The model under review builds one solid part; all positions refer to its coordinate system, in mm. Coordinates: 2 decimals unless noted, no trailing zeros. Write each loop counter-clockwise with the first axis right and the second up, starting at its lowest first coordinate (ties: lowest second). Pieces come first, ordered by that corner, then holes. Notation, with made-up numbers: (1, -16.75) - (18, -16.75) arc R12 ccw to (18, 5.25) - close; hole circle Ø9 at (49.25, -11.75). An arc over 180 degrees is marked (long way). Put each result on its own line as item: value.
Autodesk Fusion 360 part; units mm, degrees
sketch "Sketch1" plane through (0, 0, 0) normal (0, 1, 0) x (1, 0, 0)
  line L0 (7.9, 2.9) -> (7.9, 4.9)
  line L1 (-2.7515, -3.6) -> (-4.9, -5.7485)
  line L2 (2.9, -7.9) -> (4.9, -7.9)
  line L3 (-2.9, -7.9) -> (-2.9, -10.1)
  arc A0 (-10.1, -9) -> (-9, -10.1) centre (-9, -9) ccw
  line L4 (5.7485, 4.9) -> (3.6, 2.7515)
  line L5 (-7.9, 2.9) -> (-10.1, 2.9)
  line L6 (-4.9, -7.9) -> (-2.9, -7.9)
  line L7 (4.9, 5.7485) -> (4.9, 7.9)
  line L8 (10.1, 2.9) -> (7.9, 2.9)
  line L9 (9, -10.1) -> (2.9, -10.1)
  arc A1 (9, -10.1) -> (10.1, -9) centre (9, -9) ccw
  line L10 (4.9, -5.7485) -> (2.7515, -3.6)
  line L11 (5.7485, -4.9) -> (7.9, -4.9)
  line L12 (-10.1, 2.9) -> (-10.1, 9)
  line L13 (7.9, -2.9) -> (10.1, -2.9)
  line L14 (-3.6, 2.7515) -> (-5.7485, 4.9)
  line L15 (10.1, -2.9) -> (10.1, -9)
  line L16 (-2.9, 10.1) -> (-2.9, 7.9)
  line L17 (7.9, -4.9) -> (7.9, -2.9)
  line L18 (-3.6, -2.7515) -> (-3.6, 2.7515)
  line L19 (3.6, 2.7515) -> (3.6, -2.7515)
  line L20 (2.7515, -3.6) -> (-2.7515, -3.6)
  line L21 (-10.1, -9) -> (-10.1, -2.9)
  line L22 (10.1, 9) -> (10.1, 2.9)
  line L23 (2.9, 7.9) -> (2.9, 10.1)
  line L24 (7.9, 4.9) -> (5.7485, 4.9)
  line L25 (-2.9, -10.1) -> (-9, -10.1)
  line L26 (-2.7515, 3.6) -> (2.7515, 3.6)
  arc A2 (-9, 10.1) -> (-10.1, 9) centre (-9, 9) ccw
  line L27 (4.9, 7.9) -> (2.9, 7.9)
  line L28 (-7.9, -4.9) -> (-5.7485, -4.9)
  line L29 (2.9, 10.1) -> (9, 10.1)
  arc A3 (10.1, 9) -> (9, 10.1) centre (9, 9) ccw
  line L30 (-4.9, -5.7485) -> (-4.9, -7.9)
  line L31 (-7.9, -2.9) -> (-7.9, -4.9)
  line L32 (-4.9, 7.9) -> (-4.9, 5.7485)
  line L33 (2.7515, 3.6) -> (4.9, 5.7485)
  line L34 (-4.9, 5.7485) -> (-2.7515, 3.6)
  line L35 (-10.1, -2.9) -> (-7.9, -2.9)
  line L36 (3.6, -2.7515) -> (5.7485, -4.9)
  line L37 (4.9, -7.9) -> (4.9, -5.7485)
  line L38 (2.9, -10.1) -> (2.9, -7.9)
  line L39 (-5.7485, -4.9) -> (-3.6, -2.7515)
  line L40 (-7.9, 4.9) -> (-7.9, 2.9)
  line L41 (-2.9, 7.9) -> (-4.9, 7.9)
  line L42 (-9, 10.1) -> (-2.9, 10.1)
  line L43 (-5.7485, 4.9) -> (-7.9, 4.9)
  line L44 (-15.1, -14.6) -> (13.1, -14.6)
  line L45 (13.1, -14.6) -> (13.1, 14.6)
  line L46 (13.1, 14.6) -> (-15.1, 14.6)
  line L47 (-15.1, 14.6) -> (-15.1, -14.6)
  dimension "d1" = 3
  dimension "d2" = 5
  dimension "d3" = 4.5
  dimension "d4" = 4.5
extrude "Extrude1" add sketch "Sketch1" along normal blind 3 contours L0 L1 L2 L3 A0 L4 L5 L6 L7 L8 L9 A1 L10 L11 L12 L13 L14 L15 L16 L17 L18 L19 L20 L21 L22 L23 L24 L25 L26 A2 L27 L28 L29 A3 L30 L31 L32 L33 L34 L35 L36 L37 L38 L39 L40 L41 L42 L43 | L44 L45 L46 L47
extrude "Extrude2" add sketch "Sketch1" along normal blind 30 from surface at 3
mirror "Mirror1" about plane through (-15.1, 3, -14.6) normal (-1, 0, 0) of bodies 1 merged
ref_plane "WorkPlane1" through (-15.1, 16.5, -44.6) normal (0, 0, -1) x (-1, 0, 0)
sketch "Sketch2" plane through (0, 0, -44.6) normal (0, 0, -1) x (-1, 0, 0)
  line L0 (-13.1, 0) -> (43.3, 0)
  line L1 (43.3, 0) -> (43.3, 33)
  line L2 (43.3, 33) -> (-13.1, 33)
  line L3 (-13.1, 33) -> (-13.1, 0)
  line L4 (28.1, 33) -> (2.1, 33)
  line L5 (2.1, 33) -> (2.1, 7)
  line L6 (2.1, 7) -> (28.1, 7)
  line L7 (28.1, 7) -> (28.1, 33)
  line L8 (15.1, 33) -> (15.1, 0) construction
  line L9 (25.3, 30.2) -> (4.9, 30.2)
  line L10 (4.9, 30.2) -> (4.9, 9.8)
  line L11 (4.9, 9.8) -> (25.3, 9.8)
  line L12 (25.3, 9.8) -> (25.3, 30.2)
  dimension "d15" = 20.4
  dimension "d17" = 2.8
  dimension "d18" = 2.8
  dimension "d29" = 2.8
loft "Loft1" add profiles "Sketch2" section 1 face at (-5.7, 11, -14.6) section 2 contours L2 L4 L5 L6 L7 | L9 L10 L11 L12
extrude "Extrude3" cut sketch "Sketch2" against normal blind 30 contours L9 L10 L11 L12
sketch "Sketch3" plane through (0, 33, 0) normal (0, 1, 0) x (-1, 0, 0)
  line L0 (21.2, 10.1) -> (27.3, 10.1)
  line L1 (27.3, 10.1) -> (27.3, 7.9)
  line L2 (27.3, 7.9) -> (25.3, 7.9)
  line L3 (25.3, 7.9) -> (25.3, 5.7485)
  line L4 (25.3, 5.7485) -> (27.4485, 3.6)
  line L5 (27.4485, 3.6) -> (32.9515, 3.6)
  line L6 (32.9515, 3.6) -> (35.1, 5.7485)
  line L7 (35.1, 5.7485) -> (35.1, 7.9)
  line L8 (35.1, 7.9) -> (33.1, 7.9)
  line L9 (33.1, 7.9) -> (33.1, 10.1)
  line L10 (33.1, 10.1) -> (39.2, 10.1)
  arc A0 (40.3, 9) -> (39.2, 10.1) centre (39.2, 9) ccw
  line L11 (40.3, 9) -> (40.3, 2.9)
  line L12 (40.3, 2.9) -> (38.1, 2.9)
  line L13 (38.1, 2.9) -> (38.1, 4.9)
  line L14 (38.1, 4.9) -> (35.9485, 4.9)
  line L15 (35.9485, 4.9) -> (33.8, 2.7515)
  line L16 (33.8, 2.7515) -> (33.8, -2.7515)
  line L17 (33.8, -2.7515) -> (35.9485, -4.9)
  line L18 (35.9485, -4.9) -> (38.1, -4.9)
  line L19 (38.1, -4.9) -> (38.1, -2.9)
  line L20 (38.1, -2.9) -> (40.3, -2.9)
  line L21 (40.3, -2.9) -> (40.3, -9)
  arc A1 (39.2, -10.1) -> (40.3, -9) centre (39.2, -9) ccw
  line L22 (39.2, -10.1) -> (33.1, -10.1)
  line L23 (33.1, -10.1) -> (33.1, -7.9)
  line L24 (33.1, -7.9) -> (35.1, -7.9)
  line L25 (35.1, -7.9) -> (35.1, -5.7485)
  line L26 (35.1, -5.7485) -> (32.9515, -3.6)
  line L27 (32.9515, -3.6) -> (27.4485, -3.6)
  line L28 (27.4485, -3.6) -> (25.3, -5.7485)
  line L29 (25.3, -5.7485) -> (25.3, -7.9)
  line L30 (25.3, -7.9) -> (27.3, -7.9)
  line L31 (27.3, -7.9) -> (27.3, -10.1)
  line L32 (27.3, -10.1) -> (21.2, -10.1)
  arc A2 (20.1, -9) -> (21.2, -10.1) centre (21.2, -9) ccw
  line L33 (20.1, -9) -> (20.1, -2.9)
  line L34 (20.1, -2.9) -> (22.3, -2.9)
  line L35 (22.3, -2.9) -> (22.3, -4.9)
  line L36 (22.3, -4.9) -> (24.4515, -4.9)
  line L37 (24.4515, -4.9) -> (26.6, -2.7515)
  line L38 (26.6, -2.7515) -> (26.6, 2.7515)
  line L39 (26.6, 2.7515) -> (24.4515, 4.9)
  line L40 (24.4515, 4.9) -> (22.3, 4.9)
  line L41 (22.3, 4.9) -> (22.3, 2.9)
  line L42 (22.3, 2.9) -> (20.1, 2.9)
  line L43 (20.1, 2.9) -> (20.1, 9)
  arc A3 (21.2, 10.1) -> (20.1, 9) centre (21.2, 9) ccw
  line L44 (2.9, 10.1) -> (9, 10.1)
  arc A4 (10.1, 9) -> (9, 10.1) centre (9, 9) ccw
  line L45 (10.1, 9) -> (10.1, 2.9)
  line L46 (10.1, 2.9) -> (7.9, 2.9)
  line L47 (7.9, 2.9) -> (7.9, 4.9)
  line L48 (7.9, 4.9) -> (5.7485, 4.9)
  line L49 (5.7485, 4.9) -> (3.6, 2.7515)
  line L50 (3.6, 2.7515) -> (3.6, -2.7515)
  line L51 (3.6, -2.7515) -> (5.7485, -4.9)
  line L52 (5.7485, -4.9) -> (7.9, -4.9)
  line L53 (7.9, -4.9) -> (7.9, -2.9)
  line L54 (7.9, -2.9) -> (10.1, -2.9)
  line L55 (10.1, -2.9) -> (10.1, -9)
  arc A5 (9, -10.1) -> (10.1, -9) centre (9, -9) ccw
  line L56 (9, -10.1) -> (2.9, -10.1)
  line L57 (2.9, -10.1) -> (2.9, -7.9)
  line L58 (2.9, -7.9) -> (4.9, -7.9)
  line L59 (4.9, -7.9) -> (4.9, -5.7485)
  line L60 (4.9, -5.7485) -> (2.7515, -3.6)
  line L61 (2.7515, -3.6) -> (-2.7515, -3.6)
  line L62 (-2.7515, -3.6) -> (-4.9, -5.7485)
  line L63 (-4.9, -5.7485) -> (-4.9, -7.9)
  line L64 (-4.9, -7.9) -> (-2.9, -7.9)
  line L65 (-2.9, -7.9) -> (-2.9, -10.1)
  line L66 (-2.9, -10.1) -> (-9, -10.1)
  arc A6 (-10.1, -9) -> (-9, -10.1) centre (-9, -9) ccw
  line L67 (-10.1, -9) -> (-10.1, -2.9)
  line L68 (-10.1, -2.9) -> (-7.9, -2.9)
  line L69 (-7.9, -2.9) -> (-7.9, -4.9)
  line L70 (-7.9, -4.9) -> (-5.7485, -4.9)
  line L71 (-5.7485, -4.9) -> (-3.6, -2.7515)
  line L72 (-3.6, -2.7515) -> (-3.6, 2.7515)
  line L73 (-3.6, 2.7515) -> (-5.7485, 4.9)
  line L74 (-5.7485, 4.9) -> (-7.9, 4.9)
  line L75 (-7.9, 4.9) -> (-7.9, 2.9)
  line L76 (-7.9, 2.9) -> (-10.1, 2.9)
  line L77 (-10.1, 2.9) -> (-10.1, 9)
  arc A7 (-9, 10.1) -> (-10.1, 9) centre (-9, 9) ccw
  line L78 (-9, 10.1) -> (-2.9, 10.1)
  line L79 (-2.9, 10.1) -> (-2.9, 7.9)
  line L80 (-2.9, 7.9) -> (-4.9, 7.9)
  line L81 (-4.9, 7.9) -> (-4.9, 5.7485)
  line L82 (-4.9, 5.7485) -> (-2.7515, 3.6)
  line L83 (-2.7515, 3.6) -> (2.7515, 3.6)
  line L84 (2.7515, 3.6) -> (4.9, 5.7485)
  line L85 (4.9, 5.7485) -> (4.9, 7.9)
  line L86 (4.9, 7.9) -> (2.9, 7.9)
  line L87 (2.9, 7.9) -> (2.9, 10.1)
  line L88 (43.3, -14.6) -> (43.3, 14.6)
  line L89 (43.3, 14.6) -> (-13.1, 14.6)
  line L90 (-13.1, 14.6) -> (-13.1, -14.6)
  line L91 (-13.1, -14.6) -> (2.1, -44.6)
  line L92 (2.1, -44.6) -> (28.1, -44.6)
  line L93 (28.1, -44.6) -> (43.3, -14.6)
  line L94 (15.1, -44.6) -> (15.1, -17.6132) construction
  circle A8 centre (15.1, -37.1) radius 2
  circle A9 centre (15.1, -22.1) radius 2
  dimension "d23" = 4
  dimension "d24" = 7.5
  dimension "d25" = 15
extrude "Extrude4" cut sketch "Sketch3" against normal blind 4 contours A8 | A9
equation "d15 = 20 mm + 2 * gap"
equation "d17 = 3 mm - gap"
equation "d18 = 3 mm - gap"
equation "gap = 0.2 mm"
equation "d29 = 3 mm - gap"
1. To check wall thickness, follow probe 1 along Z at (x, y) = (-15, 31); probe 2 along X at (y, z) = (28.5, 0.5); probe 3 along Z at (x, y) = (-34.5, 13). State the ranges of each line that lie inside material, in increasing order.
Determined:
probe 1: z = -44.6 to -39.1, -35.1 to -24.1, -20.1 to 14.6
probe 2: x = -43.3 to -33.8, -26.6 to -3.6, 3.6 to 13.1
probe 3: z = -31.97 to -10.1, -7.9 to -5.15, -3.45 to 3.45, 5.15 to 7.9, 10.1 to 14.6
2. Consider section A-A on z = 0.5. State the section outline as (x, y) points.
Determined:
outline: (-43.3, 0) - (13.1, 0) - (13.1, 33) - (3.6, 33) - (3.6, 3) - (-3.6, 3) - (-3.6, 33) - (-26.6, 33) - (-26.6, 3) - (-33.8, 3) - (-33.8, 33) - (-43.3, 33) - close
3. For pin 1 Ø4 at (y, z) = (10.5, -17) entering from -X; pin 2 Ø0.6 at (x, y) = (4, 23) entering from -Z; pin 3 Ø4 at (x, y) = (-30.5, 7) entering from -Z, all flat-tipped, find the tip position at first contact; note any pin that passes through.
Determined:
pin 1: stops at x = -43.1
pin 2: stops at z = -33.15
pin 3: stops at z = -43.81
4. The part is to be moulded in two halves that separate along X. For faces 1 (the flat face through (4.69, 17.79, -3.84)), 2 (the flat face through (-9, 18, -2.9)), 3 (the flat face through (-4, 21, -44.6)), say which applies: +X half, -X half, draft (parallel to the pull), parting line (faces both ways), or undercut.
Determined:
face 1: undercut
face 2: undercut
face 3: draft
5. Consider section B-B on y = 12. Give the number of separate pieces and of enclosed holes in the cut face, plus the area to 3 significant figures.
Determined:
separate pieces: 1
enclosed holes: 2
area: 1,860 mm^2
